Input: part model. Units: mm. Frame: model coordinates. Coordinates: 2 decimals unless noted, no trailing zeros. Order: outer loops, then holes, each group sorted by start corner. A loop starts at its lowest first (then second) coordinate and runs counter-clockwise, first axis right, second up.
from build123d import *

# Parameters (mm, degrees)
F1_DEPTH = 50.8
F2_DEPTH = 12.7
F3_DEPTH = 25.4
F4_DEPTH = 19.05
F5_DEPTH = 3.175


with BuildPart() as f1:
    # F0 (on Top) → F1 (new body)
    with BuildSketch(Plane.XY):
        with BuildLine():
            ThreePointArc((97.792826, 81.028163), (119.475288, 43.065712), (127, 0))
            Line((127, 0), (132.08, 0))
            ThreePointArc((132.08, 0), (94.988487, 94.988487), (0, 132.08))
            Line((0, 132.08), (0, 127))
            ThreePointArc((0, 127), (19.273228, 125.529051), (38.1, 121.150279))
            ThreePointArc((38.1, 121.150279), (70.846038, 105.40322), (97.792826, 81.028163))
        make_face()
        with BuildLine():
            Line((0, 127), (0, 132.08))
            ThreePointArc((0, 132.08), (-94.988487, 94.988487), (-132.08, 0))
            Line((-132.08, 0), (-127, 0))
            ThreePointArc((-127, 0), (-119.475288, 43.065712), (-97.792826, 81.028163))
            ThreePointArc((-97.792826, 81.028163), (-70.846038, 105.40322), (-38.1, 121.150279))
            ThreePointArc((-38.1, 121.150279), (-19.273228, 125.529051), (0, 127))
        make_face()
        with BuildLine():
            Line((132.08, 0), (127, 0))
            ThreePointArc((127, 0), (120.842224, -39.066058), (102.966034, -74.343768))
            ThreePointArc((102.966034, -74.343768), (57.824482, -113.07223), (0, -127))
            Line((0, -127), (0, -132.08))
            ThreePointArc((0, -132.08), (94.988487, -94.988487), (132.08, 0))
        make_face()
        with BuildLine():
            Line((0, -132.08), (0, -127))
            ThreePointArc((0, -127), (-57.824482, -113.07223), (-102.966034, -74.343768))
            ThreePointArc((-102.966034, -74.343768), (-120.842224, -39.066058), (-127, 0))
            Line((-127, 0), (-132.08, 0))
            ThreePointArc((-132.08, 0), (-94.988487, -94.988487), (0, -132.08))
        make_face()
    extrude(amount=F1_DEPTH)

    # F0 (on Top) → F2 (join)
    with BuildSketch(Plane.XY):
        with BuildLine():
            ThreePointArc((58.165355, 52.637639), (53.045829, 88.332878), (38.1, 121.150279))
            ThreePointArc((38.1, 121.150279), (19.273228, 125.529051), (0, 127))
            ThreePointArc((0, 127), (-19.273228, 125.529051), (-38.1, 121.150279))
            ThreePointArc((-38.1, 121.150279), (-53.045829, 88.332878), (-58.165355, 52.637639))
            ThreePointArc((-58.165355, 52.637639), (-53.045829, 16.942401), (-38.1, -15.875))
            ThreePointArc((-38.1, -15.875), (-21.38592, -29.418708), (0, -31.75))
            ThreePointArc((0, -31.75), (21.38592, -29.418708), (38.1, -15.875))
            ThreePointArc((38.1, -15.875), (53.045829, 16.942401), (58.165355, 52.637639))
        make_face()
    extrude(amount=F2_DEPTH)

    # F0 (on Top) → F3 (join)
    with BuildSketch(Plane.XY):
        with BuildLine():
            ThreePointArc((0, -127), (57.824482, -113.07223), (102.966034, -74.343768))
            ThreePointArc((102.966034, -74.343768), (96.231727, -51.530394), (81.764056, -32.649519))
            ThreePointArc((81.764056, -32.649519), (61.48768, -20.212899), (38.1, -15.875))
            ThreePointArc((38.1, -15.875), (21.38592, -29.418708), (0, -31.75))
            ThreePointArc((0, -31.75), (-21.38592, -29.418708), (-38.1, -15.875))
            ThreePointArc((-38.1, -15.875), (-61.48768, -20.212899), (-81.764056, -32.649519))
            ThreePointArc((-81.764056, -32.649519), (-96.231727, -51.530394), (-102.966034, -74.343768))
            ThreePointArc((-102.966034, -74.343768), (-57.824482, -113.07223), (0, -127))
        make_face()
    extrude(amount=F3_DEPTH)

    # F0 (on Top) → F4 (join)
    with BuildSketch(Plane.XY):
        with BuildLine():
            ThreePointArc((-97.792826, 81.028163), (-119.475288, 43.065712), (-127, 0))
            ThreePointArc((-127, 0), (-111.491203, -26.174529), (-81.764056, -32.649519))
            ThreePointArc((-81.764056, -32.649519), (-61.48768, -20.212899), (-38.1, -15.875))
            ThreePointArc((-38.1, -15.875), (-53.045829, 16.942401), (-58.165355, 52.637639))
            ThreePointArc((-58.165355, 52.637639), (-83.113803, 59.665873), (-97.792826, 81.028163))
        make_face()
        with BuildLine():
            ThreePointArc((81.764056, -32.649519), (111.491203, -26.174529), (127, 0))
            ThreePointArc((127, 0), (119.475288, 43.065712), (97.792826, 81.028163))
            ThreePointArc((97.792826, 81.028163), (83.113803, 59.665873), (58.165355, 52.637639))
            ThreePointArc((58.165355, 52.637639), (53.045829, 16.942401), (38.1, -15.875))
            ThreePointArc((38.1, -15.875), (61.48768, -20.212899), (81.764056, -32.649519))
        make_face()
    extrude(amount=F4_DEPTH)

    # F0 (on Top) → F5 (join)
    with BuildSketch(Plane.XY):
        with BuildLine():
            ThreePointArc((58.165355, 52.637639), (83.113803, 59.665873), (97.792826, 81.028163))
            ThreePointArc((97.792826, 81.028163), (70.846038, 105.40322), (38.1, 121.150279))
            ThreePointArc((38.1, 121.150279), (53.045829, 88.332878), (58.165355, 52.637639))
        make_face()
        with BuildLine():
            ThreePointArc((102.966034, -74.343768), (120.842224, -39.066058), (127, 0))
            ThreePointArc((127, 0), (111.491203, -26.174529), (81.764056, -32.649519))
            ThreePointArc((81.764056, -32.649519), (96.231727, -51.530394), (102.966034, -74.343768))
        make_face()
        with BuildLine():
            ThreePointArc((-127, 0), (-120.842224, -39.066058), (-102.966034, -74.343768))
            ThreePointArc((-102.966034, -74.343768), (-96.231727, -51.530394), (-81.764056, -32.649519))
            ThreePointArc((-81.764056, -32.649519), (-111.491203, -26.174529), (-127, 0))
        make_face()
        with BuildLine():
            ThreePointArc((-58.165355, 52.637639), (-53.045829, 88.332878), (-38.1, 121.150279))
            ThreePointArc((-38.1, 121.150279), (-70.846038, 105.40322), (-97.792826, 81.028163))
            ThreePointArc((-97.792826, 81.028163), (-83.113803, 59.665873), (-58.165355, 52.637639))
        make_face()
    extrude(amount=F5_DEPTH)


solid = f1.part
Item 1: Pin query (flat end, axial travel): pin 1 Ø4 at (x, z) = (66.5, 43) entering from -Y; pin 2 Ø4 at (y, z) = (-36, 45) entering from -X; pin 3 Ø13.5 at (x, y) = (-115, -19) entering from +Z; pin 4 Ø3 at (x, y) = (24, 68.5) entering from -Z. Return the tip coordinate at first contact, or that it passes through.
Response values:
pin 1: stops at y = -117.48
pin 2: stops at x = -128.87
pin 3: stops at z = 19.05
pin 4: stops at z = 0
Item 2: Cut plane D-D on y = 116.5. Return loops of the section in (x, z) (3 decimals).
Response values:
outline: (-66.327, 0) - (66.327, 0) - (66.327, 50.8) - (50.564, 50.8) - (50.564, 3.175) - (40.941, 3.175) - (40.941, 12.7) - (-40.941, 12.7) - (-40.941, 3.175) - (-50.564, 3.175) - (-50.564, 50.8) - (-66.327, 50.8) - close
Item 3: Ray query, probe 1 along X at (y, z) = (-8.5, 6); probe 2 along X at (y, z) = (-72, 4); probe 3 along Z at (x, y) = (-87.5, -58.5). Return the intervals inside material, ascending.
Response values:
probe 1: x = -132.14 to -126.72, -124.93 to 124.93, 126.72 to 132.14
probe 2: x = -113.19 to -104.62, -102.68 to 102.68, 104.62 to 113.19
probe 3: z = 0 to 25.4
Item 4: Draft query along Y for faces 1 (the face through (83.41, 59.88, 11)), 2 (the face through (-2, 2, 0)). Return one class per face: pulls with the +Y half, pulls with the -Y half, needs draft (parallel to the pull), parting line crosses it, or undercut.
Response values:
face 1: undercut
face 2: needs draft
Item 5: Cut plane B-B on z = 9.5. Return loops of the section in (x, y).
Response values:
outline: (-132.08, 0) arc R127 ccw to (0, -132.08) arc R127 ccw to (132.08, 0) arc R127 ccw to (0, 132.08) arc R127 ccw to start; hole (-127, 0) arc R127 ccw to (-102.97, -74.34) arc R65.22 cw to (-81.76, -32.65) arc R38.1 cw to start; hole (-97.79, 81.03) arc R38.1 ccw to (-58.17, 52.64) arc R127 cw to (-38.1, 121.15) arc R127 ccw to start; hole (38.1, 121.15) arc R127 cw to (58.17, 52.64) arc R38.1 ccw to (97.79, 81.03) arc R127 ccw to start; hole (81.76, -32.65) arc R65.22 cw to (102.97, -74.34) arc R127 ccw to (127, 0) arc R38.1 cw to start
Item 6: Cut plane A-A on z = 31. Return loops of the section in (x, y).
Response values:
outline: (-132.08, 0) arc R127 ccw to (0, -132.08) arc R127 ccw to (132.08, 0) arc R127 ccw to (0, 132.08) arc R127 ccw to start; hole (-102.97, -74.34) arc R127 ccw to (0, -127) arc R127 ccw to (102.97, -74.34) arc R127 ccw to (97.79, 81.03) arc R127 ccw to (38.1, 121.15) arc R127 ccw to (0, 127) arc R127 ccw to (-38.1, 121.15) arc R127 ccw to (-97.79, 81.03) arc R127 ccw to start
Item 7: Cut plane C-C on x = 21. Return loops of the section in (y, z), then the cut area to 3 significant figures.
Response values:
outline: (-131.2, 0) - (131.2, 0) - (131.2, 50.8) - (125.25, 50.8) - (125.25, 12.7) - (-29.58, 12.7) - (-29.58, 25.4) - (-125.25, 25.4) - (-125.25, 50.8) - (-131.2, 50.8) - close
area: 5,000 mm2
